Source: CAD feature listing. Evaluate the final solid. Frame: model axes, mm. A direction names the side the tool comes from. Round coordinates to 2 decimals unless told otherwise and drop trailing zeros. Write each loop counter-clockwise with the first axis right and the second up, starting at its lowest first coordinate (ties: lowest second). Pieces come first, ordered by that corner, then holes.
from build123d import *

# Parameters (mm, degrees)
F0_W      = 131.572
F0_H      = 80.772
F0_W_2    = 127
F0_H_2    = 76.2
F1_DEPTH  = 25.4
F1_FACE_W = 131.572
F1_FACE_H = 25.4
F3_DEPTH  = 2.032
F2_W      = 126.530789
F2_H      = 75.769949
F4_DEPTH  = 2.032


with BuildPart() as f1:
    # F0 (on Top) → F1 (new body)
    with BuildSketch(Plane.XY):
        Rectangle(F0_W, F0_H)
        Rectangle(F0_W_2, F0_H_2, mode=Mode.SUBTRACT)
    extrude(amount=F1_DEPTH)

    # F1_face (on face) → F3 (join)
    with BuildSketch(Plane(origin=(0, -40.386, 12.7), x_dir=(1, 0, 0), z_dir=(0, -1, 0))):
        Rectangle(F1_FACE_W, F1_FACE_H)
    extrude(amount=F3_DEPTH)

    # F2 (on Top) → F4 (join)
    with BuildSketch(Plane.XY):
        with Locations((0.215594, -0.227573)):
            Rectangle(F2_W, F2_H)
    extrude(amount=F4_DEPTH)


solid = f1.part
1) Section query B-B on z = 3.5. Return the cut outline in (x, y).
Taken from the geometry:
outline: (-65.79, -42.42) - (65.79, -42.42) - (65.79, 40.39) - (-65.79, 40.39) - close; hole (-63.5, -38.1) - (63.5, -38.1) - (63.5, 38.1) - (-63.5, 38.1) - close
2) Section query A-A on x = -48.5. Return the cut outline in (y, z), then the cut area to 3 significant figures.
Taken from the geometry:
outline: (-42.42, 0) - (37.66, 0) - (37.66, 2.03) - (-38.1, 2.03) - (-38.1, 25.4) - (-42.42, 25.4) - close; (38.1, 0) - (40.39, 0) - (40.39, 25.4) - (38.1, 25.4) - close
area: 322 mm2
3) Pull-direction query (X, two-part tool) for faces 4 (the face through (-20, -41, 25.4)), 5 (the face through (-1, -38.1, 15)), 6 (the face through (65.786, 0, 13)); classes: released by +X, released by -X, zero draft, split by the parting line, or undercut.
Taken from the geometry:
face 4: zero draft
face 5: undercut
face 6: released by +X
4) Material intervals for line 1 (Y direction, x = 35.5, z = 11.5); line 2 (X direction, y = -33, z = 13.5); line 3 (Z direction, x = 58.5, y = -2), sorted ascending.
Taken from the geometry:
line 1: y = -42.42 to -38.1, 38.1 to 40.39
line 2: x = -65.79 to -63.5, 63.5 to 65.79
line 3: z = 0 to 2.03
5) Section query C-C on y = -17. Return the cut outline in (x, z), then the cut area to 3 significant figures.
Taken from the geometry:
outline: (-65.79, 0) - (-63.5, 0) - (-63.5, 25.4) - (-65.79, 25.4) - close; (-63.05, 0) - (63.48, 0) - (63.48, 2.03) - (-63.05, 2.03) - close; (63.5, 0) - (65.79, 0) - (65.79, 25.4) - (63.5, 25.4) - close
area: 373 mm2
6) Reachability of faces 1 (the face through (-1, -42.418, 13)), 2 (the face through (-63.5, -1, 13)), 3 (the face through (-1, 0, 2.032)) from +Z, -Z, +X, -X, +Y, -Y: full face, straight path, thin tool, end or side. Return the list, or none.
Taken from the geometry:
face 1: +Z, -Z, +X, -X, -Y
face 2: +Z, -Z
face 3: +Z
